from build123d import *

# Parameters (mm, degrees)
SKETCH1_W           = 8.2
SKETCH1_H           = 8.2
SKETCH1_W_2         = 5.2
SKETCH1_H_2         = 5.2
BOSS_EXTRUDE1_DEPTH = 20
SKETCH2_W           = 8.2
SKETCH2_H           = 8.2
BOSS_EXTRUDE2_DEPTH = 20
SHELL1_T            = -1.5


with BuildPart() as part:
    # Sketch1 → Boss-Extrude1 (new body)
    # profile 1 of 2: a face of its own
    with BuildSketch(Plane(origin=(0, 0, 0), x_dir=(1, 0, 0), z_dir=(0, 1, 0))):
        Rectangle(SKETCH1_W, SKETCH1_H)
        Rectangle(SKETCH1_W_2, SKETCH1_H_2, mode=Mode.SUBTRACT)
    # profile 2 of 2: a face of its own
    with BuildSketch(Plane(origin=(0, 0, 0), x_dir=(1, 0, 0), z_dir=(0, 1, 0))):
        Rectangle(SKETCH1_W_2, SKETCH1_H_2)
    extrude(amount=BOSS_EXTRUDE1_DEPTH)

    # Sketch2 → Boss-Extrude2 (add)
    with BuildSketch(Plane(origin=(0, 0, 4.1), x_dir=(-1, 0, 0), z_dir=(0, 0, -1))):
        with Locations((0, 4.1)):
            Rectangle(SKETCH2_W, SKETCH2_H)
    extrude(amount=BOSS_EXTRUDE2_DEPTH)

    # Shell1
    shell1_openings = [part.faces().sort_by_distance(p)[0] for p in [
        (0, 20, 0),
        (0, 4.1, -15.9),
    ]]
    offset(amount=SHELL1_T, openings=shell1_openings, kind=Kind.INTERSECTION)


solid = part.part
Can you work these out from the model? Positions are in its coordinate system, mm. A direction names the side the tool comes from. Round coordinates to 2 decimals unless told otherwise and drop trailing zeros. Loops run counter-clockwise (first coordinate to the right, second up) from the corner with the lowest first, then second, coordinate; pieces in that order, holes last. Notation, with made-up numbers: (70.5, 3.25) - (101.5, 3.25) arc R24 cw to (101.5, 26.25) - close; hole circle Ø6 at (-27.5, 80). An arc over 180 degrees is marked (long way). Write item = value, one per line. Start each with the question number.
(1) If we section it at B-B (z = -3): Please give me the cut outline in (x, y), and give its area (3 significant figures).
(2) If I drill on probe 1 along Z at (x, y) = (2.5, 9); probe 2 along Y at (x, z) = (1, -10.25), over which ranges is the centre line in solid material (lowest first)? Write a range as [from, to].
(3) If we section it at C-C (y = 7.75): Please give me the cut outline in (x, z).
(4) If we section it at A-A (x = 2.25): Please give me the cut outline in (y, z), and give its area (3 significant figures).
(5) For P1, Ø1, axis at x = -3, z = -6.5, coming from the +Y side; P2, Ø4, axis at x = 0.5, y = 12, coming from the -Z side, each with a flat end and sliding along its axis, tell me the tip position at first contact or that it passes through.
(6) If we mould it in two halves opening along Z, with no side actions, what happens to faces 1 (the face through (0, 1.5, -7)), 2 (the face through (3, 4, -15.9)), 3 (the face through (0, 11, 2.6))? For each: released by +Z, released by -Z, zero draft, split by the parting line, or undercut.
(7) For faces 4 (the face through (0, 14, -4.1)), 5 (the face through (0, 6.7, -9)), 6 (the face through (-2.6, 6.5, -4.5)), 7 (the face through (0, 13, -2.6)), which set-ups out of +Z, -Z, +X, -X, +Y, -Y let a thin tool reach every point of the face, with its end or its side?
(8) If we section it at D-D (y = 2.5): Please give me the cut outline in (x, z), and give its area (3 significant figures).
Ans:
q1.outline = (-4.1, 0) - (4.1, 0) - (4.1, 20) - (-4.1, 20) - close; hole (-2.6, 1.5) - (2.6, 1.5) - (2.6, 6.7) - (-2.6, 6.7) - close
q1.area = 137 mm²
q2.probe_1 = [-4.1, -2.6], [2.6, 4.1]
q2.probe_2 = [0, 1.5], [6.7, 8.2]
q3.outline = (-4.1, -15.9) - (4.1, -15.9) - (4.1, 4.1) - (-4.1, 4.1) - close; hole (-2.6, -2.6) - (2.6, -2.6) - (2.6, 2.6) - (-2.6, 2.6) - close
q4.outline = (0, -15.9) - (1.5, -15.9) - (1.5, 2.6) - (20, 2.6) - (20, 4.1) - (0, 4.1) - close; (6.7, -15.9) - (8.2, -15.9) - (8.2, -4.1) - (20, -4.1) - (20, -2.6) - (6.7, -2.6) - close
q4.area = 95.4 mm²
q5.P1 = 8.2
q5.P2 = -4.1
q6.face_1 = zero draft
q6.face_2 = released by -Z
q6.face_3 = undercut
q7.face_4 = -Z, +X, -X, +Y
q7.face_5 = -Z
q7.face_6 = none
q7.face_7 = +Y
q8.outline = (-4.1, -15.9) - (-2.6, -15.9) - (-2.6, 2.6) - (2.6, 2.6) - (2.6, -15.9) - (4.1, -15.9) - (4.1, 4.1) - (-4.1, 4.1) - close
q8.area = 67.8 mm²
